from build123d import *

# Parameters (mm, degrees)
SKETCH1_R           = 17.5
SKETCH1_R_2         = 11
BOSS_EXTRUDE1_DEPTH = 3.5
SKETCH4_R           = 4
CUT_EXTRUDE1_DEPTH  = 6.8
CIRPATTERN1_COUNT   = 8


with BuildPart() as part:
    # Sketch1 → Boss-Extrude1 (new body, symmetric)
    with BuildSketch(Plane.XY):
        Circle(SKETCH1_R)
        Circle(SKETCH1_R_2, mode=Mode.SUBTRACT)
    extrude(amount=BOSS_EXTRUDE1_DEPTH, both=True)

    # Sketch4 → Cut-Extrude1 (cut)
    with BuildSketch(Plane(origin=(-10.162674858, 0, 0), x_dir=(0, 0, -1), z_dir=(1, 0, 0))):
        Circle(SKETCH4_R)
    cut_extrude1 = extrude(amount=-CUT_EXTRUDE1_DEPTH, mode=Mode.SUBTRACT)

    # CirPattern1: Cut-Extrude1 ×8 about axis
    cirpattern1_axis = Axis((0, 0, 0), (0, 0, 1))
    for i in range(1, CIRPATTERN1_COUNT):
        add(cut_extrude1.rotate(cirpattern1_axis, i * 360 / CIRPATTERN1_COUNT), mode=Mode.SUBTRACT)


solid = part.part
CAD build for the part. Positions are in the model's coordinates, mm. A direction names the side the tool comes from. Coordinates: 2 decimals unless noted, no trailing zeros. Write each loop counter-clockwise with the first axis right and the second up, starting at its lowest first coordinate (ties: lowest second). Pieces come first, ordered by that corner, then holes. Notation, with made-up numbers: (-19.75, 77.5) - (8.25, 77.5) arc R19 cw to (8.25, 92.5) - close; hole circle Ø2 at (22, 8). An arc over 180 degrees is marked (long way). Use a Markdown table: item, result. Add a question column.
Item 1: Drill centre lines: L1, parallel to Y at x = -11, z = -3; L2, parallel to X at y = 10.5, z = -0.5; L3, parallel to X at y = 11, z = 0.75. Where is each one in solid material? Low to high. Write a range as from..to.
Item 2: Flat gauge pin, fed straight in: pin 1 (3 mm diameter, centred on x = -13, z = -1.5, fed in from +Y). Where does the tip first touch, or does it go through?
Item 3: Band-saw the part on A-A, the plane y = 0. Give the cut face in (x, z).
Item 4: 3-axis set-ups, long thin cutter, end or side, ignore diameter. For faces 5 (the face through (10.167, 4.199, 0.243)), 6 (the face through (3, -12, 3.5)), 7 (the face through (14, 4, 0)): which of +Z, -Z, +X, -X, +Y, -Y reach the whole face in a straight line?
Item 5: Mould opens along Z. For faces 1 (the face through (3, -12, -3.5)), 2 (the face through (12.034, 11.955, 0.049)), 3 (the face through (-4, 14, 0)), 4 (the face through (-13.887, -10.648, 0.049)) say: pulls with the +Z half, pulls with the -Z half, needs draft (parallel to the pull), parting line crosses it, or undercut.
Numbers:
| question | item | result |
|---|---|---|
| 1 | L1 | -13.61..-12.99, -7.26..-2.65, 2.65..7.26, 12.99..13.61 |
| 1 | L2 | -14..-13.49, -4.89..-3.97, 3.97..4.89, 13.49..14 |
| 1 | L3 | -13.61..-12.99, -5.44..-3.93, 3.93..5.44, 12.99..13.61 |
| 2 | pin 1 | y = 13.19 |
| 3 | outline | (-17.5, -3.5) - (-16.96, -3.5) - (-16.96, 3.5) - (-17.5, 3.5) - close; (16.96, -3.5) - (17.5, -3.5) - (17.5, 3.5) - (16.96, 3.5) - close |
| 4 | face 5 | +Z, -Z |
| 4 | face 6 | +Z, +X, -X, +Y, -Y |
| 4 | face 7 | none |
| 5 | face 1 | pulls with the -Z half |
| 5 | face 2 | undercut |
| 5 | face 3 | undercut |
| 5 | face 4 | needs draft |
